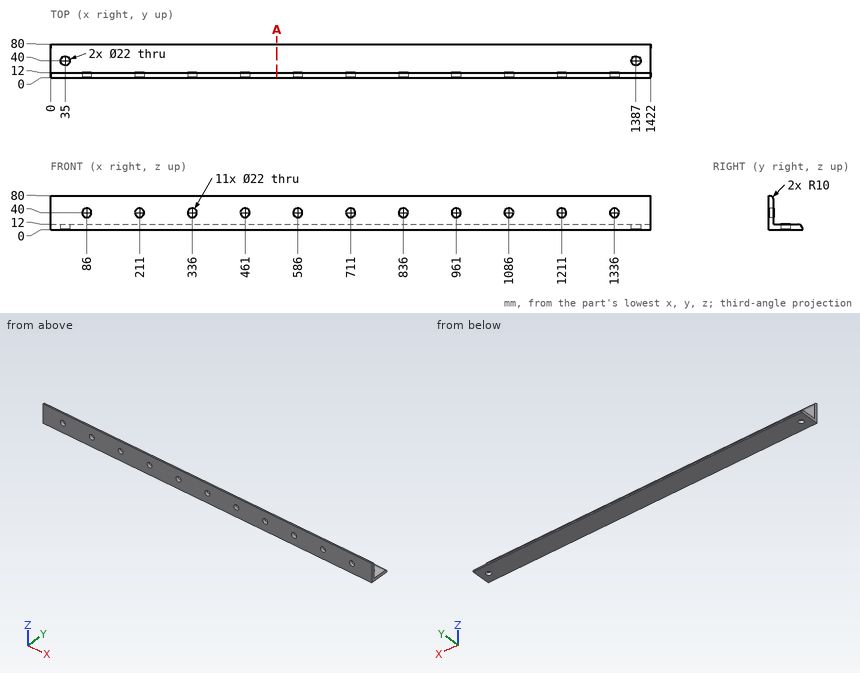
Here's the drawing with two shaded views (mm, measured from the low corner). I have some questions. Round coordinates to 2 decimals unless told otherwise and drop trailing zeros. Loops run counter-clockwise (first coordinate to the right, second up) from the corner with the lowest first, then second, coordinate; pieces in that order, holes last.
1. Suppose I cut it at A-A, the plane x = 536.5. Please give me the cut outline in (y, z), and give its area (3 significant figures).
Answers:
outline: (0, 0) - (80, 0) - (80, 2) arc R10 ccw to (70, 12) - (12, 12) - (12, 70) arc R10 ccw to (2, 80) - (0, 80) - close
area: 1,730 mm2
2. If I drill on probe 1 along X at (y, z) = (41, 8); probe 2 along Z at (x, y) = (836, 4.25); probe 3 along Z at (x, y) = (1107.5, 38), over which ranges is the centre line in solid material (lowest first)?
Answers:
probe 1: x = 0 to 24.05, 45.95 to 1376.05, 1397.95 to 1422
probe 2: z = 0 to 29, 51 to 79.74
probe 3: z = 0 to 12
3. Will these pins go through, and if not, where does the flat tip stop? pin 1 (17.5 mm diameter, centred on x = 461, z = 40, fed in from +Y); pin 2 (1 mm diameter, centred on x = 861, y = 64, fed in from +Z); pin 3 (2 mm diameter, centred on x = 513, z = 21, fed in from +Y).
Answers:
pin 1: passes through
pin 2: stops at z = 12
pin 3: stops at y = 12
